Geometry: final body of the model. Coordinates: model frame, mm. Face numbers are marked on the shaded views. A direction names the side the tool comes from. Round coordinates to 2 decimals unless told otherwise and drop trailing zeros. Order: outer loops, then holes, each group sorted by start corner. A loop starts at its lowest first (then second) coordinate and runs counter-clockwise, first axis right, second up. Notation, with made-up numbers: (80.5, -32) -> (127.5, -32) arc R22 cw to (127.5, -4) -> close; hole circle Ø7 at (35, -8). An arc over 180 degrees is marked (long way). Put each result on its own line as item: value.
```python
from build123d import *

# Parameters (mm, degrees)
F0_R         = 5.25
F1_DEPTH     = 8
F2_R         = 32
F2_R_2       = 22
F3_DEPTH     = 30
F4_T4_ANGLE  = 106.1070017135
F4_T9_ANGLE  = 106.1070017135
F4_T15_ANGLE = 106.1070017135
F4_T20_ANGLE = 106.1070017135
F4_T25_ANGLE = 106.1070017135
F4_T31_ANGLE = 106.1070017135
F4_T36_ANGLE = 106.1070017135
F4_T41_ANGLE = 106.1070017135
F4_T47_ANGLE = 106.1070017135
F4_T52_ANGLE = 106.1070017135
F4_T57_ANGLE = 106.1070017135
F4_T63_ANGLE = 106.1070017135
F5_R         = 5
F6_DEPTH     = 19.3


# Not quite as in the source:
# - a fillet or chamfer that OpenCascade refuses, or shapes differently, is made with other operations: its cross-section is extruded or revolved along the edge and cut away or added


with BuildPart() as f1:
    # F0 (on Top) → F1 (new body)
    with BuildSketch(Plane.XY):
        with BuildLine():
            ThreePointArc((3, 31.8590646441), (22.627416998, 22.627416998), (31.8590646441, 3))
            Line((31.8590646441, 3), (63.4290942707, 3))
            ThreePointArc((63.4290942707, 3), (44.9012806053, 44.9012806053), (3, 63.4290942707))
            Line((3, 63.4290942707), (3, 31.8590646441))
        make_face()
        with Locations((30.7591449816, 30.7591449816)):
            Circle(F0_R, mode=Mode.SUBTRACT)
        with BuildLine():
            ThreePointArc((-31.8590646441, 3), (-22.627416998, 22.627416998), (-3, 31.8590646441))
            Line((-3, 31.8590646441), (-3, 63.4290942707))
            ThreePointArc((-3, 63.4290942707), (-44.9012806053, 44.9012806053), (-63.4290942707, 3))
            Line((-63.4290942707, 3), (-31.8590646441, 3))
        make_face()
        with Locations((-30.7591449816, 30.7591449816)):
            Circle(F0_R, mode=Mode.SUBTRACT)
        with BuildLine():
            Line((-3, -63.4290942707), (-3, -31.8590646441))
            ThreePointArc((-3, -31.8590646441), (-22.627416998, -22.627416998), (-31.8590646441, -3))
            Line((-31.8590646441, -3), (-63.4290942707, -3))
            ThreePointArc((-63.4290942707, -3), (-44.9012806053, -44.9012806053), (-3, -63.4290942707))
        make_face()
        with Locations((-30.7591449816, -30.7591449816)):
            Circle(F0_R, mode=Mode.SUBTRACT)
        with BuildLine():
            Line((63.4290942707, -3), (31.8590646441, -3))
            ThreePointArc((31.8590646441, -3), (22.627416998, -22.627416998), (3, -31.8590646441))
            Line((3, -31.8590646441), (3, -63.4290942707))
            ThreePointArc((3, -63.4290942707), (44.9012806053, -44.9012806053), (63.4290942707, -3))
        make_face()
        with Locations((30.7591449816, -30.7591449816)):
            Circle(F0_R, mode=Mode.SUBTRACT)
        with BuildLine():
            ThreePointArc((31.8590646441, -3), (31.9647467424, -1.501654319), (32, 0))
            ThreePointArc((32, 0), (31.9647467424, 1.501654319), (31.8590646441, 3))
            ThreePointArc((31.8590646441, 3), (22.627416998, 22.627416998), (3, 31.8590646441))
            ThreePointArc((3, 31.8590646441), (0, 32), (-3, 31.8590646441))
            ThreePointArc((-3, 31.8590646441), (-22.627416998, 22.627416998), (-31.8590646441, 3))
            ThreePointArc((-31.8590646441, 3), (-32, 0), (-31.8590646441, -3))
            ThreePointArc((-31.8590646441, -3), (-22.627416998, -22.627416998), (-3, -31.8590646441))
            ThreePointArc((-3, -31.8590646441), (0, -32), (3, -31.8590646441))
            ThreePointArc((3, -31.8590646441), (22.627416998, -22.627416998), (31.8590646441, -3))
        make_face()
    extrude(amount=F1_DEPTH)

    # F2 (on face) → F3 (join)
    with BuildSketch(Plane.XY.offset(8)):
        Circle(F2_R)
        Circle(F2_R_2, mode=Mode.SUBTRACT)
    extrude(amount=F3_DEPTH)

    # F4: fillet of radius 3 on 6 edges, made by hand


with BuildPart() as f4_tool2:
    # F4_s3 → F4_t4 (revolve)
    with BuildSketch(Plane(origin=(0, 0, 0), x_dir=(0, 0, 1), z_dir=(-0.1400977189, -0.9901376819, 0))):
        with BuildLine():
            ThreePointArc((11, -32), (8.8786796564, -32.8786796564), (8, -35))
            Line((8, -35), (8, -32))
            Line((8, -32), (11, -32))
        make_face()
    revolve(axis=Axis((0, 0, 8), (0, 0, 1)), revolution_arc=F4_T4_ANGLE)

    split(bisect_by=Plane.XZ.offset(3), keep=Keep.TOP)


with BuildPart() as f1_1:
    add(f1.part)

    # F4_t1: union F4_tool2
    add(f4_tool2.part)


with BuildPart() as f4_tool7:
    # F4_s8 → F4_t9 (revolve)
    with BuildSketch(Plane(origin=(0, 0, 0), x_dir=(0, 0, 1), z_dir=(-0.1400977189, -0.9901376819, 0))):
        with BuildLine():
            ThreePointArc((11, -32), (8.8786796564, -32.8786796564), (8, -35))
            Line((8, -35), (8, -32))
            Line((8, -32), (11, -32))
        make_face()
    revolve(axis=Axis((0, 0, 8), (0, 0, 1)), revolution_arc=F4_T9_ANGLE)

    split(bisect_by=Plane.YZ.offset(3), keep=Keep.TOP)

    split(bisect_by=Plane.XZ.offset(-3), keep=Keep.BOTTOM)


with BuildPart() as f1_2:
    add(f1_1.part)

    # F4_t6: union F4_tool7
    add(f4_tool7.part)


with BuildPart() as f4_tool13:
    # F4_s14 → F4_t15 (revolve)
    with BuildSketch(Plane(origin=(0, 0, 0), x_dir=(0, 0, 1), z_dir=(-0.1400977189, -0.9901376819, 0))):
        with BuildLine():
            ThreePointArc((11, -32), (8.8786796564, -32.8786796564), (8, -35))
            Line((8, -35), (8, -32))
            Line((8, -32), (11, -32))
        make_face()
    revolve(axis=Axis((0, 0, 8), (0, 0, 1)), revolution_arc=F4_T15_ANGLE)

    split(bisect_by=Plane.YZ.offset(-3), keep=Keep.BOTTOM)


with BuildPart() as f1_3:
    add(f1_2.part)

    # F4_t12: union F4_tool13
    add(f4_tool13.part)


with BuildPart() as f4_tool18:
    # F4_s19 → F4_t20 (revolve)
    with BuildSketch(Plane(origin=(0, 0, 0), x_dir=(0, 0, 1), z_dir=(-0.9901376819, 0.1400977189, 0))):
        with BuildLine():
            ThreePointArc((11, -32), (8.8786796564, -32.8786796564), (8, -35))
            Line((8, -35), (8, -32))
            Line((8, -32), (11, -32))
        make_face()
    revolve(axis=Axis((0, 0, 8), (0, 0, 1)), revolution_arc=F4_T20_ANGLE)

    split(bisect_by=Plane.YZ.offset(-3), keep=Keep.BOTTOM)


with BuildPart() as f1_4:
    add(f1_3.part)

    # F4_t17: union F4_tool18
    add(f4_tool18.part)


with BuildPart() as f4_tool23:
    # F4_s24 → F4_t25 (revolve)
    with BuildSketch(Plane(origin=(0, 0, 0), x_dir=(0, 0, 1), z_dir=(-0.9901376819, 0.1400977189, 0))):
        with BuildLine():
            ThreePointArc((11, -32), (8.8786796564, -32.8786796564), (8, -35))
            Line((8, -35), (8, -32))
            Line((8, -32), (11, -32))
        make_face()
    revolve(axis=Axis((0, 0, 8), (0, 0, 1)), revolution_arc=F4_T25_ANGLE)

    split(bisect_by=Plane.XZ.offset(3), keep=Keep.TOP)

    split(bisect_by=Plane.YZ.offset(3), keep=Keep.TOP)


with BuildPart() as f1_5:
    add(f1_4.part)

    # F4_t22: union F4_tool23
    add(f4_tool23.part)


with BuildPart() as f4_tool29:
    # F4_s30 → F4_t31 (revolve)
    with BuildSketch(Plane(origin=(0, 0, 0), x_dir=(0, 0, 1), z_dir=(-0.9901376819, 0.1400977189, 0))):
        with BuildLine():
            ThreePointArc((11, -32), (8.8786796564, -32.8786796564), (8, -35))
            Line((8, -35), (8, -32))
            Line((8, -32), (11, -32))
        make_face()
    revolve(axis=Axis((0, 0, 8), (0, 0, 1)), revolution_arc=F4_T31_ANGLE)

    split(bisect_by=Plane.XZ.offset(-3), keep=Keep.BOTTOM)


with BuildPart() as f1_6:
    add(f1_5.part)

    # F4_t28: union F4_tool29
    add(f4_tool29.part)


with BuildPart() as f4_tool34:
    # F4_s35 → F4_t36 (revolve)
    with BuildSketch(Plane(origin=(0, 0, 0), x_dir=(0, 0, 1), z_dir=(0.1400977189, 0.9901376819, 0))):
        with BuildLine():
            ThreePointArc((11, -32), (8.8786796564, -32.8786796564), (8, -35))
            Line((8, -35), (8, -32))
            Line((8, -32), (11, -32))
        make_face()
    revolve(axis=Axis((0, 0, 8), (0, 0, 1)), revolution_arc=F4_T36_ANGLE)

    split(bisect_by=Plane.XZ.offset(-3), keep=Keep.BOTTOM)


with BuildPart() as f1_7:
    add(f1_6.part)

    # F4_t33: union F4_tool34
    add(f4_tool34.part)


with BuildPart() as f4_tool39:
    # F4_s40 → F4_t41 (revolve)
    with BuildSketch(Plane(origin=(0, 0, 0), x_dir=(0, 0, 1), z_dir=(0.1400977189, 0.9901376819, 0))):
        with BuildLine():
            ThreePointArc((11, -32), (8.8786796564, -32.8786796564), (8, -35))
            Line((8, -35), (8, -32))
            Line((8, -32), (11, -32))
        make_face()
    revolve(axis=Axis((0, 0, 8), (0, 0, 1)), revolution_arc=F4_T41_ANGLE)

    split(bisect_by=Plane.XZ.offset(3), keep=Keep.TOP)

    split(bisect_by=Plane.YZ.offset(-3), keep=Keep.BOTTOM)


with BuildPart() as f1_8:
    add(f1_7.part)

    # F4_t38: union F4_tool39
    add(f4_tool39.part)


with BuildPart() as f4_tool45:
    # F4_s46 → F4_t47 (revolve)
    with BuildSketch(Plane(origin=(0, 0, 0), x_dir=(0, 0, 1), z_dir=(0.1400977189, 0.9901376819, 0))):
        with BuildLine():
            ThreePointArc((11, -32), (8.8786796564, -32.8786796564), (8, -35))
            Line((8, -35), (8, -32))
            Line((8, -32), (11, -32))
        make_face()
    revolve(axis=Axis((0, 0, 8), (0, 0, 1)), revolution_arc=F4_T47_ANGLE)

    split(bisect_by=Plane.YZ.offset(3), keep=Keep.TOP)


with BuildPart() as f1_9:
    add(f1_8.part)

    # F4_t44: union F4_tool45
    add(f4_tool45.part)


with BuildPart() as f4_tool50:
    # F4_s51 → F4_t52 (revolve)
    with BuildSketch(Plane(origin=(0, 0, 0), x_dir=(0, 0, 1), z_dir=(0.9901376819, -0.1400977189, 0))):
        with BuildLine():
            ThreePointArc((11, -32), (8.8786796564, -32.8786796564), (8, -35))
            Line((8, -35), (8, -32))
            Line((8, -32), (11, -32))
        make_face()
    revolve(axis=Axis((0, 0, 8), (0, 0, 1)), revolution_arc=F4_T52_ANGLE)

    split(bisect_by=Plane.YZ.offset(3), keep=Keep.TOP)


with BuildPart() as f1_10:
    add(f1_9.part)

    # F4_t49: union F4_tool50
    add(f4_tool50.part)


with BuildPart() as f4_tool55:
    # F4_s56 → F4_t57 (revolve)
    with BuildSketch(Plane(origin=(0, 0, 0), x_dir=(0, 0, 1), z_dir=(0.9901376819, -0.1400977189, 0))):
        with BuildLine():
            ThreePointArc((11, -32), (8.8786796564, -32.8786796564), (8, -35))
            Line((8, -35), (8, -32))
            Line((8, -32), (11, -32))
        make_face()
    revolve(axis=Axis((0, 0, 8), (0, 0, 1)), revolution_arc=F4_T57_ANGLE)

    split(bisect_by=Plane.XZ.offset(-3), keep=Keep.BOTTOM)

    split(bisect_by=Plane.YZ.offset(-3), keep=Keep.BOTTOM)


with BuildPart() as f1_11:
    add(f1_10.part)

    # F4_t54: union F4_tool55
    add(f4_tool55.part)


with BuildPart() as f4_tool61:
    # F4_s62 → F4_t63 (revolve)
    with BuildSketch(Plane(origin=(0, 0, 0), x_dir=(0, 0, 1), z_dir=(0.9901376819, -0.1400977189, 0))):
        with BuildLine():
            ThreePointArc((11, -32), (8.8786796564, -32.8786796564), (8, -35))
            Line((8, -35), (8, -32))
            Line((8, -32), (11, -32))
        make_face()
    revolve(axis=Axis((0, 0, 8), (0, 0, 1)), revolution_arc=F4_T63_ANGLE)

    split(bisect_by=Plane.XZ.offset(3), keep=Keep.TOP)


with BuildPart() as f1_12:
    add(f1_11.part)

    # F4_t60: union F4_tool61
    add(f4_tool61.part)

    # F5 (on face) → F6 (cut)
    with BuildSketch(Plane.XY.offset(8)):
        Circle(F5_R)
    extrude(amount=-F6_DEPTH, mode=Mode.SUBTRACT)


solid = f1_12.part
```
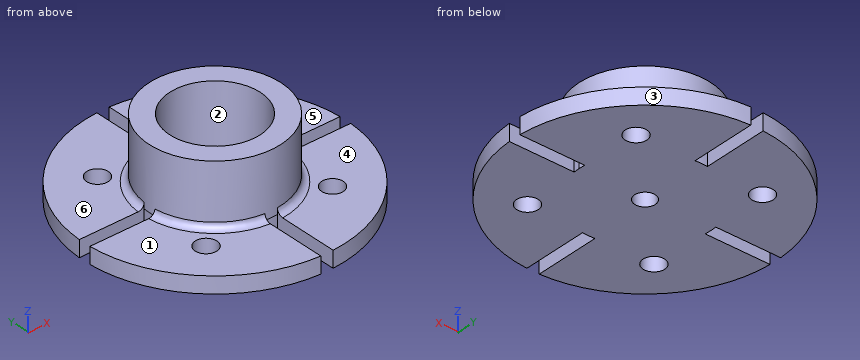
1. Cut plane C-C on z = 21.5. Return loops of the section in (x, y), and give its area (3 significant figures).
Ans:
outline: circle Ø64 at (0, 0); hole circle Ø44 at (0, 0)
area: 1,700 mm²
2. Contact query for flat-ended pins moving along their axis: P1, Ø18, axis at x = 37, y = 43.5, coming from the +Z side; P2, Ø4, axis at x = -27, z = 19, coming from the -Y side (3 decimals); P3, Ø9, axis at y = -46, z = 4.5, coming from the +X side. Output: stop coordinate, or through.
Ans:
P1: z = 8
P2: y = -19.975
P3: x = 48.06
3. Cut plane B-B on y = 48. Return loops of the section in (x, z), and give its area (3 significant figures).
Ans:
outline: (-41.57, 0) -> (-3, 0) -> (-3, 8) -> (-41.57, 8) -> close; (3, 0) -> (41.57, 0) -> (41.57, 8) -> (3, 8) -> close
area: 617 mm²
4. Cut plane A-A on x = 0. Return loops of the section in (y, z).
Ans:
outline: (-32, 0) -> (-5, 0) -> (-5, 8) -> (-22, 8) -> (-22, 38) -> (-32, 38) -> close; (5, 0) -> (32, 0) -> (32, 38) -> (22, 38) -> (22, 8) -> (5, 8) -> close
5. Set-up query: the marked faces 4, 5 and 6. Return all of +Z, -Z, +X, -X, +Y, -Y with unobstructed straight access to the full face (end or side cutting, diameter ignored); none if empty.
Ans:
face 4: +Z, +X, -Y
face 5: +Z, +X, +Y
face 6: +Z, -X, +Y
6. Draft query along X for the marked faces 1, 2 and 3. Return one class per face: +X half, -X half, draft (parallel to the pull), parting line (faces both ways), or undercut.
Ans:
face 1: draft
face 2: undercut
face 3: +X half
7. Material intervals for probe 1 along Y at (x, z) = (27.5, 7.5); probe 2 along X at (y, z) = (2.5, 13); probe 3 along X at (y, z) = (9.5, 17), sorted ascending.
Ans:
probe 1: -57.24 to -34.88, -26.64 to 26.64, 34.88 to 57.24
probe 2: -31.9 to -21.86, 21.86 to 31.9
probe 3: -30.56 to -19.84, 19.84 to 30.56
